For this review, take the finished solid that the model builds, in its own axes (mm). Round coordinates to 2 decimals unless told otherwise and drop trailing zeros. Order: outer loops, then holes, each group sorted by start corner. A loop starts at its lowest first (then second) coordinate and runs counter-clockwise, first axis right, second up. Notation, with made-up numbers: M 2,35 L 46,35 A16 cw 46,64 Z; hole C -33,88 d2. An arc over 180 degrees is marked long. Answer in a Markdown table with one row per item. Add a question column.
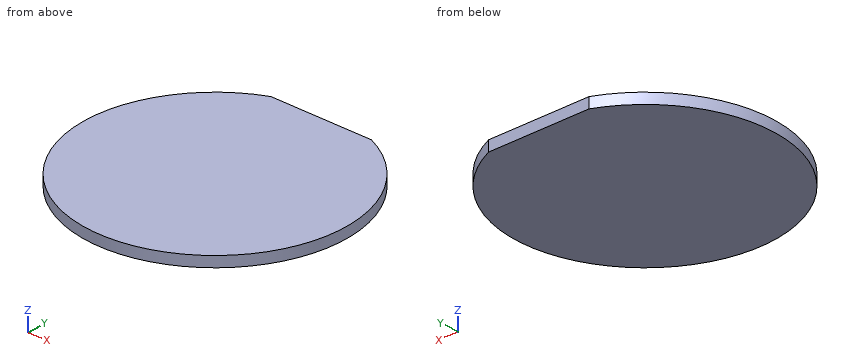
```python
from build123d import *

# Parameters (mm, degrees)
BOX818_W           = 148
BOX818_H           = 20
BOX818_DEPTH       = 34
CYLINDER1864_R     = 74
CYLINDER1864_DEPTH = 6


with BuildPart() as krychle818:
    # Box818 → Box818 (new body)
    with BuildSketch(Plane(origin=(-74, 68, 38), x_dir=(1, 0, 0), z_dir=(0, 0, 1))):
        with Locations((74, 10)):
            Rectangle(BOX818_W, BOX818_H)
    extrude(amount=BOX818_DEPTH)


with BuildPart() as cut603:
    # Cylinder1864 → Cylinder1864 (new body)
    with BuildSketch(Plane.XY.offset(65)):
        Circle(CYLINDER1864_R)
    extrude(amount=CYLINDER1864_DEPTH)

    # Cut603: cut Krychle818
    add(krychle818.part, mode=Mode.SUBTRACT)


with BuildPart() as cut603_1:
    # Cut603 placement: moved
    add(cut603.part.moved(Location((0, 0, 13))))


solid = cut603_1.part
```
1. Consider section B-B on x = 33. Write out the cut boundary in (y, z), plus the area to 3 significant figures.
2. To check wall thickness, follow probe 1 along Y at (x, z) = (68, 83.6); probe 2 along Y at (x, z) = (10, 78.8). State the ranges of each line that lie inside material, in increasing order. Write a range as [from, to].
3. Clearance check with a flat-ended pin moving along its axis: pin 1 Ø2 at (y, z) = (18, 83) entering from +X. State where the tip first meets the part, or that it passes through.
4. Consider section A-A on z = 80.6. Write out the cut boundary in (x, y), plus the area to 3 significant figures.
5. Consider section C-C on y = -42. Write out the cut boundary in (x, z), plus the area to 3 significant figures.
Solved:
| question | item | result |
|---|---|---|
| 1 | outline | M -66.23,78 L 66.23,78 L 66.23,84 L -66.23,84 Z |
| 1 | area | 795 mm^2 |
| 2 | probe 1 | y = [-29.19, 29.19] |
| 2 | probe 2 | y = [-73.32, 68] |
| 3 | pin 1 | stops at x = 72.02 |
| 4 | outline | M -29.19,68 A74 ccw long 29.19,68 Z |
| 4 | area | 17,000 mm^2 |
| 5 | outline | M -60.93,78 L 60.93,78 L 60.93,84 L -60.93,84 Z |
| 5 | area | 731 mm^2 |
